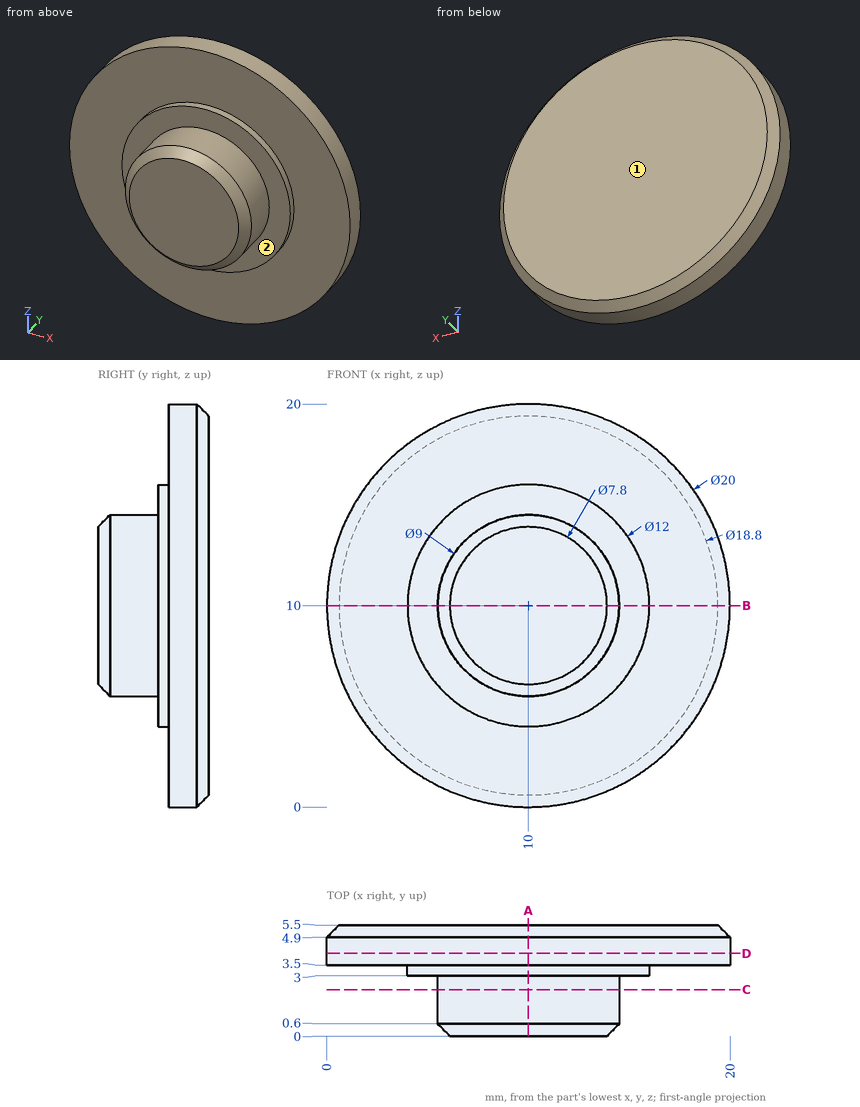
The drawing under review shows one solid part. Ordinate dimensions are in mm from its lowest x, y, z. A direction names the side the tool comes from. Give positions to 0.01 mm unless a question says otherwise; leave off trailing zeros. Write each loop counter-clockwise with the first axis right and the second up, starting at its lowest first coordinate (ties: lowest second). Pieces come first, ordered by that corner, then holes. Notation, with made-up numbers: (-11, 50.5) - (9, 50.5) arc R34 cw to (9, 86.5) - close; hole circle Ø1 at (-29, 12). An arc over 180 degrees is marked (long way). Answer in a Markdown table with one row per item. Add a question column.
1. We need section B-B on z = 10. Write out the cut boundary in (x, y).
2. Wall thickness on line 1 along Y through (x, z) = (11.5, 3.75); line 2 along X through (y, z) = (1.95, 7.75); line 3 along X through (y, z) = (4.7, 17.25): over which ranges is each line inside the solid? List them lowest first. Write a range as [from, to].
3. Tool access review of the marked faces 1 and 2: name each direction out of +Z, -Z, +X, -X, +Y, -Y from which nothing blocks a thin tool from reaching the whole face with its end or side.
4. We need section A-A on x = 10. Write out the cut boundary in (y, z), then the cut area to 3 significant figures.
5. We need section D-D on y = 4.1. Write out the cut boundary in (x, z), then the cut area to 3 significant figures.
6. Insertion check: P1, Ø3.5, axis at x = 9.5, z = 12, coming from the -Y side; P2, Ø3, axis at y = 4.5, z = 17, coming from the +X side; P3, Ø1.5, axis at x = 12, y = 2, coming from the -Z side; P4, Ø2, axis at y = 4.5, z = 18, coming from the -X side. Each pin has a flat end and moves straight along its axis. Give the tip position at first contact, or say it passes through.
7. We need section C-C on y = 2.3. Write out the cut boundary in (x, z).
Ans:
| question | item | result |
|---|---|---|
| 1 | outline | (0, 3.5) - (4, 3.5) - (4, 3) - (5.5, 3) - (5.5, 0.6) - (6.1, 0) - (13.9, 0) - (14.5, 0.6) - (14.5, 3) - (16, 3) - (16, 3.5) - (20, 3.5) - (20, 4.9) - (19.4, 5.5) - (0.6, 5.5) - (0, 4.9) - close |
| 2 | line 1 | y = [3.5, 5.5] |
| 2 | line 2 | x = [6.1, 13.9] |
| 2 | line 3 | x = [3.11, 16.89] |
| 3 | face 1 | +Z, -Z, +X, -X, +Y |
| 3 | face 2 | -Y |
| 4 | outline | (0, 6.1) - (0.6, 5.5) - (3, 5.5) - (3, 4) - (3.5, 4) - (3.5, 0) - (4.9, 0) - (5.5, 0.6) - (5.5, 19.4) - (4.9, 20) - (3.5, 20) - (3.5, 16) - (3, 16) - (3, 14.5) - (0.6, 14.5) - (0, 13.9) - close |
| 4 | area | 72.3 mm^2 |
| 5 | outline | circle Ø20 at (10, 10) |
| 5 | area | 314 mm^2 |
| 6 | P1 | stops at y = 0 |
| 6 | P2 | stops at x = 18.35 |
| 6 | P3 | stops at z = 5.68 |
| 6 | P4 | stops at x = 2.86 |
| 7 | outline | circle Ø9 at (10, 10) |
